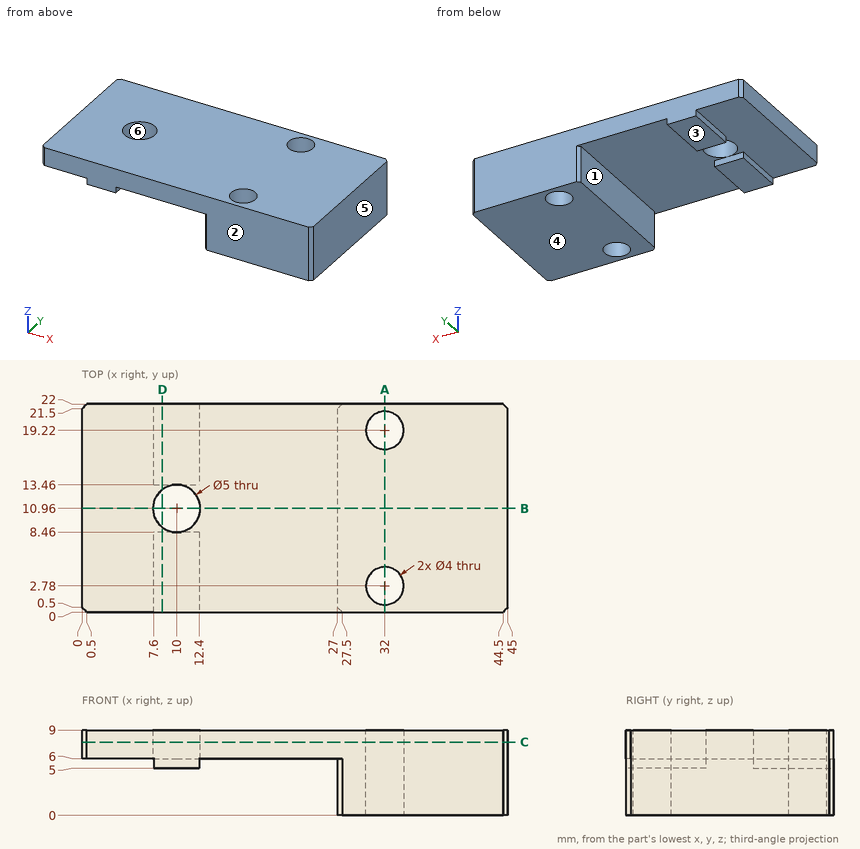
Part print with two shaded views. Sizes in mm from the minimum x, y, z corner. A direction names the side the tool comes from. Round coordinates to 2 decimals unless told otherwise and drop trailing zeros. Loops run counter-clockwise (first coordinate to the right, second up) from the corner with the lowest first, then second, coordinate; pieces in that order, holes last. Notation, with made-up numbers: (58, 18.25) - (113, 18.25) arc R23 cw to (113, 28.25) - close; hole circle Ø4 at (21.5, 52). An arc over 180 degrees is marked (long way). Answer as a JSON object with one key per item and string values.
Item 1: Band-saw the part on A-A on x = 32. List the corners of the cut face in (y, z), plus the area to 3 significant figures.
Output:
{"outline": "(0, 0) - (0.78, 0) - (0.78, 9) - (0, 9) - close; (4.78, 0) - (17.22, 0) - (17.22, 9) - (4.78, 9) - close; (21.22, 0) - (22, 0) - (22, 9) - (21.22, 9) - close", "area": "126 mm2"}
Item 2: Band-saw the part on D-D on x = 8.5. List the corners of the cut face in (y, z), plus the area to 3 significant figures.
Output:
{"outline": "(0, 5) - (8.46, 5) - (8.46, 6) - (8.96, 6) - (8.96, 9) - (0, 9) - close; (12.96, 6) - (13.46, 6) - (13.46, 5) - (22, 5) - (22, 9) - (12.96, 9) - close", "area": "71.0 mm2"}
Item 3: Band-saw the part on B-B on y = 10.96. List the corners of the cut face in (x, z), plus the area to 3 significant figures.
Output:
{"outline": "(0, 6) - (7.5, 6) - (7.5, 9) - (0, 9) - close; (12.5, 6) - (27, 6) - (27, 0) - (45, 0) - (45, 9) - (12.5, 9) - close", "area": "228 mm2"}
Item 4: Pin check, flat tips, straight feed: pin 1 (3 mm diameter, centred on x = 32, y = 2.78, fed in from +Z); pin 2 (1 mm diameter, centred on y = 15.5, z = 4, fed in from -X); pin 3 (1.1 mm diameter, centred on y = 19.5, z = 5.5, fed in from -X); pin 4 (8 mm diameter, centred on x = 4.5, y = 12.5, fed in from -Z). Stop position of each tip, or through.
Output:
{"pin 1": "through", "pin 2": "x = 27", "pin 3": "x = 0", "pin 4": "z = 5"}
Item 5: Wall check: L1, parallel to Y at x = 32, z = 3.5; L2, parallel to Y at x = 10, z = 7.55; L3, parallel to Y at x = 31, z = 4.75. Give the ranges that are in metal, low to high.
Output:
{"L1": "0 to 0.78, 4.78 to 17.22, 21.22 to 22", "L2": "0 to 8.46, 13.46 to 22", "L3": "0 to 1.05, 4.51 to 17.49, 20.95 to 22"}
Item 6: Pull direction X, two halves, no side cores. Call the marked faces 4, 5 and 6: pulls with the +X half, pulls with the -X half, needs draft (parallel to the pull), parting line crosses it, or undercut.
Output:
{"face 4": "needs draft", "face 5": "pulls with the +X half", "face 6": "undercut"}
Item 7: Band-saw the part on C-C on z = 7.75. List the corners of the cut face in (x, y).
Output:
{"outline": "(0, 0.5) - (0.5, 0) - (44.5, 0) - (45, 0.5) - (45, 21.5) - (44.5, 22) - (0.5, 22) - (0, 21.5) - close; hole circle Ø5 at (10, 10.96); hole circle Ø4 at (32, 2.78); hole circle Ø4 at (32, 19.22)"}
Item 8: Tool access for the marked faces 1, 2 and 3: list every direction of +Z, -Z, +X, -X, +Y, -Y with a clear straight run to the whole face (end or side of a thin tool).
Output:
{"face 1": "-Z, +Y, -Y", "face 2": "+Z, -Z, +X, -X, -Y", "face 3": "-Z, -X, +Y, -Y"}
